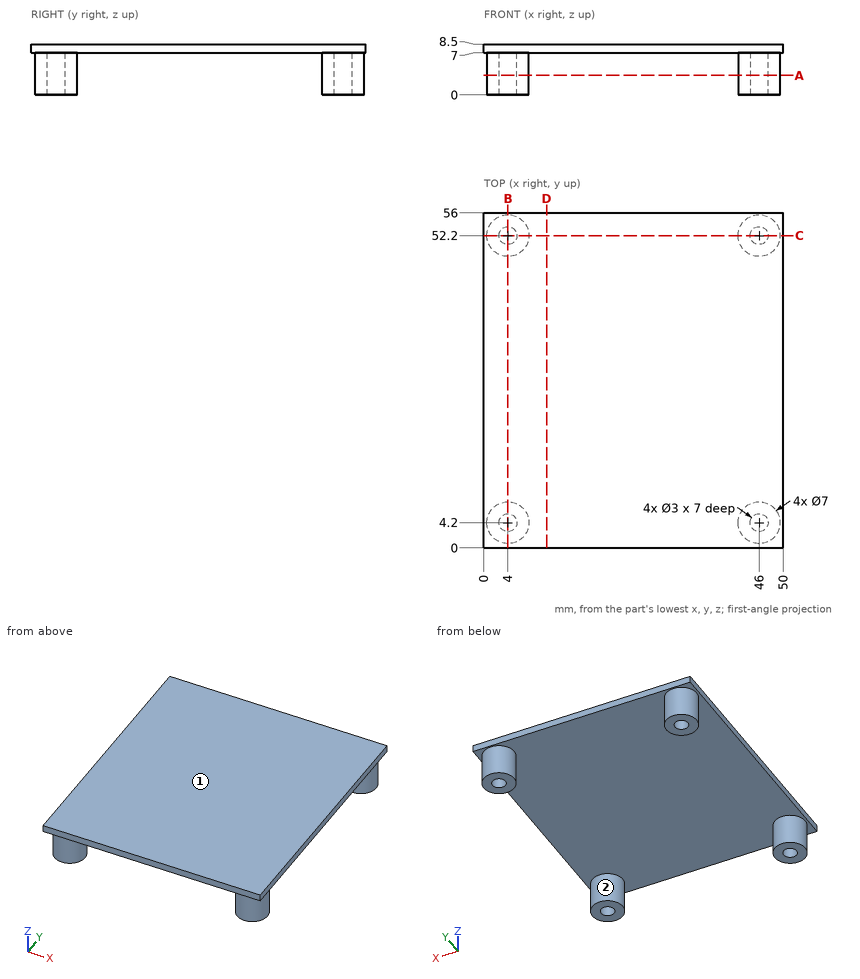
For this review, use the dimensioned drawing (mm, ordinates from the lowest corner) and the shaded views. Round coordinates to 2 decimals unless told otherwise and drop trailing zeros. Write each loop counter-clockwise with the first axis right and the second up, starting at its lowest first coordinate (ties: lowest second). Pieces come first, ordered by that corner, then holes. Notation, with made-up numbers: M -32,73 L -3,73 A27 cw -3,108 Z; hole C 3.25,78.5 d9. An arc over 180 degrees is marked long. Use CSV: the item, a comma, the result in double quotes. Start each with the question number.
(1) Clearance check with flat-ended pins moving along their axes: P1, Ø2.5, axis at x = 4.5, y = 4.5, coming from the -Z side; P2, Ø1.5, axis at x = 4.5, y = 52, coming from the -Z side; P3, Ø1.5, axis at y = 41.5, z = 5.5, coming from the +X side. State where each tip first meets the part, or that it passes through.
(2) We need section D-D, the plane x = 10.5. State the section outline as (y, z) points.
(3) For line 1 along Y through (x, z) = (4, 3); line 2 along Z through (x, y) = (31, 53); line 3 along Y through (x, z) = (43.5, 2.5), list the stretches that pass through material, from the lowest coordinate up.
(4) We need section C-C, the plane y = 52.2. State the section outline as (x, z) points.
(5) The part is to be moulded in two halves that separate along X. For the marked faces 1 and 2, say which applies: +X half, -X half, draft (parallel to the pull), parting line (faces both ways), or undercut.
(6) We need section A-A, the plane z = 3.25. State the section outline as (x, y) points, then the cut area to 3 significant figures.
(7) We need section B-B, the plane x = 4. State the section outline as (y, z) points, then the cut area to 3 significant figures.
Findings:
1,P1,"z = 0"
1,P2,"z = 7"
1,P3,"through"
2,outline,"M 0,7 L 56,7 L 56,8.5 L 0,8.5 Z"
3,line 1,"0.7 to 2.7, 5.7 to 7.7, 48.7 to 50.7, 53.7 to 55.7"
3,line 2,"7 to 8.5"
3,line 3,"1.75 to 6.65, 49.75 to 54.65"
4,outline,"M 0,7 L 0.5,7 L 0.5,0 L 2.5,0 L 2.5,7 L 5.5,7 L 5.5,0 L 7.5,0 L 7.5,7 L 42.5,7 L 42.5,0 L 44.5,0 L 44.5,7 L 47.5,7 L 47.5,0 L 49.5,0 L 49.5,7 L 50,7 L 50,8.5 L 0,8.5 Z"
5,face 1,"draft"
5,face 2,"undercut"
6,outline,"C 4,4.2 d7; C 4,52.2 d7; C 46,4.2 d7; C 46,52.2 d7; hole C 4,4.2 d3; hole C 4,52.2 d3; hole C 46,4.2 d3; hole C 46,52.2 d3"
6,area,"126 mm^2"
7,outline,"M 0,7 L 0.7,7 L 0.7,0 L 2.7,0 L 2.7,7 L 5.7,7 L 5.7,0 L 7.7,0 L 7.7,7 L 48.7,7 L 48.7,0 L 50.7,0 L 50.7,7 L 53.7,7 L 53.7,0 L 55.7,0 L 55.7,7 L 56,7 L 56,8.5 L 0,8.5 Z"
7,area,"140 mm^2"
